Input: part model. Units: mm. Frame: model coordinates. A direction names the side the tool comes from. Give positions to 0.01 mm unless a question says otherwise; leave off trailing zeros. Loops run counter-clockwise (first coordinate to the right, second up) from the corner with the lowest first, then second, coordinate; pieces in that order, holes last. Notation, with made-up numbers: M 50.25,1.5 L 108.25,1.5 A21 cw 108.25,13.5 Z; hole C 77,33.25 d11. An arc over 180 degrees is marked long. One line per item, written item: value. Start each with the question number.
(1) Section A-A on x = 6.35. Output: boundary loops of the cut face in (y, z), plus the area to 3 significant figures.
(2) Pin query (flat end, axial travel): P1, Ø3, axis at y = -20, z = -15, coming from the -X side; P2, Ø1, axis at x = 5.5, z = 18, coming from the -Y side; P3, Ø1, axis at x = 6.5, z = -12.5, coming from the -Y side; P4, Ø4, axis at x = 6.35, z = -23.2, coming from the +Y side. Return the tip coordinate at first contact, or that it passes through.
(3) Ray query, line 1 along Z through (x, y) = (7, -5); line 2 along Z through (x, y) = (6.75, -15.5); line 3 along Y through (x, z) = (5.25, -18). Return the intervals inside material, ascending. Write a range as from..to.
(4) Section B-B on y = -14. Output: boundary loops of the cut face in (x, z) (3 decimals).
(5) Access query for faces 1 (the flat face through (12.7, -18, 0)), 2 (the flat face through (3, -25.4, 25)). Directions: +Z, -Z, +X, -X, +Y, -Y. A direction counts if a zero-diameter tool reaches every point of the face in a straight line with its end or side. Return the directions, or none.
(6) Section C-C on z = -21. Output: boundary loops of the cut face in (x, y).
(7) Pull-direction query (Z, two-part tool) for faces 3 (the cylindrical face through (7.566, -12.878, -20.266)), 4 (the cylindrical face through (6.261, -17.776, -0.391)), 5 (the flat face through (5, -25.4, -20)), 6 (the cylindrical face through (6.26, -30.48, 0.25)); classes: released by +Z, released by -Z, zero draft, split by the parting line, or undercut.
(8) Section D-D on y = -20. Output: boundary loops of the cut face in (x, z) (3 decimals).
```python
from build123d import *

# Parameters (mm, degrees)
BOSS_EXTRUDE1_DEPTH = 12.7
SKETCH2_R           = 3.175
CUT_EXTRUDE1_DEPTH  = 41.982449048


with BuildPart() as part:
    # Sketch1 → Boss-Extrude1 (new body)
    with BuildSketch(Plane(origin=(0, 0, 0), x_dir=(0, 0, -1), z_dir=(1, 0, 0))):
        with BuildLine():
            Line((-17.78, 0), (-29.548453935, 0))
            Line((-29.548453935, 0), (-29.548453935, -25.4))
            Line((-29.548453935, -25.4), (-16.848453935, -25.4))
            ThreePointArc((-16.848453935, -25.4), (0, -30.48), (16.848453935, -25.4))
            Line((16.848453935, -25.4), (29.548453935, -25.4))
            Line((29.548453935, -25.4), (29.548453935, 0))
            Line((29.548453935, 0), (17.78, 0))
            ThreePointArc((17.78, 0), (0, -17.78), (-17.78, 0))
        make_face()
    extrude(amount=BOSS_EXTRUDE1_DEPTH)

    # Sketch2 → Cut-Extrude1 (cut, through all)
    with BuildSketch(Plane.XZ.offset(25.4)):
        with Locations(Location((6.35, 23.198453935, 0), (0, 0, 270))):
            Circle(SKETCH2_R)
        with Locations(Location((6.35, -23.198453935, 0), (0, 0, 90))):
            Circle(SKETCH2_R)
    extrude(amount=-CUT_EXTRUDE1_DEPTH, mode=Mode.SUBTRACT)


solid = part.part
```
Output values:
1. outline: M -25.4,-29.55 L 0,-29.55 L 0,-26.37 L -25.4,-26.37 Z; M -25.4,-20.02 L 0,-20.02 L 0,-17.78 A17.78 cw 0,17.78 L 0,20.02 L -25.4,20.02 L -25.4,16.85 A30.48 ccw -25.4,-16.85 Z; M -25.4,26.37 L 0,26.37 L 0,29.55 L -25.4,29.55 Z
1. area: 798 mm²
2. P1: stops at x = 0
2. P2: stops at y = -25.4
2. P3: stops at y = -28.02
2. P4: passes through
3. line 1: z = -29.55..-26.31, -20.09..-17.06, 17.06..20.09, 26.31..29.55
3. line 2: z = -29.55..-26.35, -20.05..-8.71, 8.71..20.05, 26.35..29.55
3. line 3: y = -25.4..0
4. outline: M 0,-29.548 L 12.7,-29.548 L 12.7,-10.96 L 0,-10.96 Z; M 0,10.96 L 12.7,10.96 L 12.7,29.548 L 0,29.548 Z; hole C 6.35,-23.198 d6.35; hole C 6.35,23.198 d6.35
5. face 1: +Z, -Z, +X, +Y, -Y
5. face 2: +Z, +X, -X, -Y
6. outline: M 0,-25.4 L 4.06,-25.4 L 4.06,0 L 0,0 Z; M 8.64,-25.4 L 12.7,-25.4 L 12.7,0 L 8.64,0 Z
7. face 3: undercut
7. face 4: undercut
7. face 5: zero draft
7. face 6: split by the parting line
8. outline: M 0,-29.548 L 12.7,-29.548 L 12.7,29.548 L 0,29.548 Z; hole C 6.35,-23.198 d6.35; hole C 6.35,23.198 d6.35
